```python
from build123d import *

# Parameters (mm, degrees)
SKETCH3_W         = 0.79
SKETCH3_H         = 3.1
SKETCH4_W         = 0.395
SKETCH4_H         = 0.395
CIRPATTERN1_COUNT = 2
CIRPATTERN1_ANGLE = 90


with BuildPart() as part:
    # BodySke → Base-Revolve (revolve)
    with BuildSketch(Plane.XY):
        Polygon((0, 0), (0, 2.75), (0.45, 2.75), (1.7, 1.5), (7, 1.5), (7, 0), align=None)
    revolve(axis=Axis((-6.35, 0, 0), (1, 0, 0)))

    # Sketch3 → Cross section 0
    with BuildSketch(Plane.ZY):
        Rectangle(SKETCH3_W, SKETCH3_H)
    # Sketch4 → Cross section 1
    with BuildSketch(Plane.ZY.offset(-2.08)):
        Rectangle(SKETCH4_W, SKETCH4_H)
    cross = loft(mode=Mode.SUBTRACT)

    # CirPattern1: Cross ×2 about axis
    cirpattern1_axis = Axis((0, 0, 0), (1, 0, 0))
    for i in range(1, CIRPATTERN1_COUNT):
        add(cross.rotate(cirpattern1_axis, i * CIRPATTERN1_ANGLE / (CIRPATTERN1_COUNT - 1)), mode=Mode.SUBTRACT)


solid = part.part
```
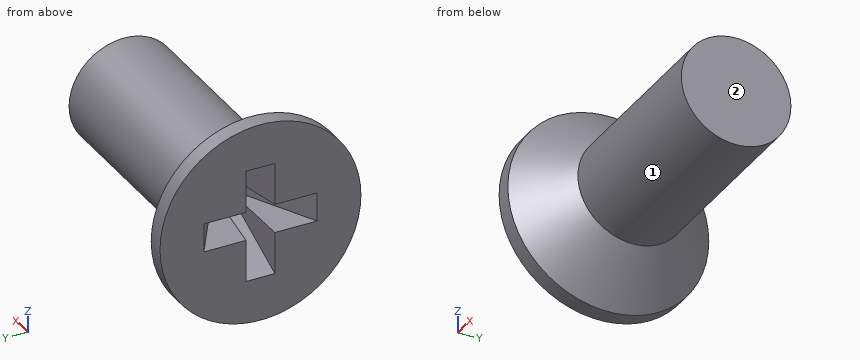
CAD build for the part. Positions are in the model's coordinates, mm. Face numbers are marked on the shaded views. A direction names the side the tool comes from. Round coordinates to 2 decimals unless told otherwise and drop trailing zeros. Order: outer loops, then holes, each group sorted by start corner. A loop starts at its lowest first (then second) coordinate and runs counter-clockwise, first axis right, second up.
Item 1: Saw through at A-A on x = 3. Write the cut outline in (y, z).
Item 2: Pin check, flat tips, straight feed: pin 1 (3 mm diameter, centred on x = 2, y = -2, fed in from +Z); pin 2 (3 mm diameter, centred on x = 5.5, y = 1.5, fed in from +Z); pin 3 (3 mm diameter, centred on x = 2, z = 0.5, fed in from -Y). Stop position of each tip, or through.
Item 3: Probe line 1 along Z through (x, y) = (1.25, -0.1); line 2 along X through (y, z) = (0.55, -2.5); line 3 along X through (y, z) = (-0.7, 0.1). List the from-to ranges inside material, lowest first.
Item 4: Tool access for the marked faces 1 and 2: list every direction of +Z, -Z, +X, -X, +Y, -Y with a clear straight run to the whole face (end or side of a thin tool).
Reported:
1. outline: circle Ø3 at (0, 0)
2. pin 1: stops at z = 2.17
2. pin 2: stops at z = 1.5
2. pin 3: stops at y = -2.67
3. line 1: z = -1.95 to -0.74, 0.74 to 1.95
3. line 2: x = 0 to 0.64
3. line 3: x = 1.31 to 7
4. face 1: +X
4. face 2: +Z, -Z, +X, +Y, -Y
